from build123d import *

# Parameters (mm, degrees)
CROQUIS2_W              = 43
CROQUIS2_H              = 30
SALIENTE_EXTRUIR1_DEPTH = 30
CROQUIS3_W              = 42.529407755
CROQUIS3_H              = 25.558495791
CORTAR_EXTRUIR1_DEPTH   = 30
CORTAR_EXTRUIR2_START   = -7.5
CORTAR_EXTRUIR2_DEPTH   = 15
CORTAR_EXTRUIR4_DEPTH   = 4.5
CORTAR_EXTRUIR5_DEPTH   = 4.5
REDONDEO1_R             = 3
CROQUIS8_W              = 15
CROQUIS8_H              = 32.397186909
CORTAR_EXTRUIR6_DEPTH   = 4.5
CROQUIS9_W              = 120.283196461
CROQUIS9_H              = 78.810135234
CORTAR_EXTRUIR7_DEPTH   = 22.5


with BuildPart() as part:
    # Croquis2 → Saliente-Extruir1 (new body)
    with BuildSketch(Plane(origin=(0, 0, 0), x_dir=(0, 0, -1), z_dir=(1, 0, 0))):
        with Locations((-19.783269962, -13.522813688)):
            Rectangle(CROQUIS2_W, CROQUIS2_H)
    extrude(amount=SALIENTE_EXTRUIR1_DEPTH)

    # Croquis3 → Cortar-Extruir1 (cut)
    with BuildSketch(Plane(origin=(30, 0, 0), x_dir=(0, 0, -1), z_dir=(1, 0, 0))):
        with Locations((-17.018566085, -31.302061584)):
            Rectangle(CROQUIS3_W, CROQUIS3_H)
        Polygon((-31.675073764, 1.477186312), (-3.283269962, -16.522813688), (1.716730038, -16.522813688), (1.716730038, 1.477186312), align=None)
    extrude(amount=-CORTAR_EXTRUIR1_DEPTH, mode=Mode.SUBTRACT)

    # Croquis4 → Cortar-Extruir2 (cut)
    with BuildSketch(Plane(origin=(30, 0, 0), x_dir=(0, 0, -1), z_dir=(1, 0, 0)).offset(CORTAR_EXTRUIR2_START)):
        Polygon((-41.283269962, -1.522813688), (-32.545919554, -1.522813688), (-8.886083053, -16.522813688), (-41.283269962, -16.522813688), align=None)
    extrude(amount=-CORTAR_EXTRUIR2_DEPTH, mode=Mode.SUBTRACT)

    # Croquis5 → Cortar-Extruir4 (cut)
    with BuildSketch(Plane(origin=(30, 0, 0), x_dir=(0, 0, -1), z_dir=(1, 0, 0))):
        Polygon((-3.283269962, -16.522813688), (-41.283269962, -16.522813688), (-41.283269962, 1.477186312), (-31.675073764, 1.477186312), align=None)
    extrude(amount=-CORTAR_EXTRUIR4_DEPTH, mode=Mode.SUBTRACT)

    # Croquis6 → Cortar-Extruir5 (cut)
    with BuildSketch(Plane.ZY):
        Polygon((3.283269962, -16.522813688), (41.283269962, -16.522813688), (41.283269962, 1.477186312), (31.675073764, 1.477186312), align=None)
    extrude(amount=-CORTAR_EXTRUIR5_DEPTH, mode=Mode.SUBTRACT)

    # Redondeo1
    redondeo1_edges = [part.edges().sort_by_distance(p)[0] for p in [
        (0, -17.522813688, -1.716730038),
        (30, -17.522813688, -1.716730038),
    ]]
    fillet(redondeo1_edges, radius=REDONDEO1_R)

    # Croquis8 → Cortar-Extruir6 (cut)
    with BuildSketch(Plane(origin=(0, -16.522813688, 0), x_dir=(1, 0, 0), z_dir=(0, 1, 0))):
        with Locations((15, -25.084676508)):
            Rectangle(CROQUIS8_W, CROQUIS8_H)
    extrude(amount=-CORTAR_EXTRUIR6_DEPTH, mode=Mode.SUBTRACT)

    # Croquis9 → Cortar-Extruir7 (cut)
    with BuildSketch(Plane.XZ.offset(18.522813688)):
        with Locations((17.6156444, 62.089659259)):
            Rectangle(CROQUIS9_W, CROQUIS9_H)
    extrude(amount=CORTAR_EXTRUIR7_DEPTH, mode=Mode.SUBTRACT)


solid = part.part
Geometry: final body of the model. Coordinates: model frame, mm. A direction names the side the tool comes from. Give positions to 0.01 mm unless a question says otherwise; leave off trailing zeros. Write each loop counter-clockwise with the first axis right and the second up, starting at its lowest first coordinate (ties: lowest second). Pieces come first, ordered by that corner, then holes. Notation, with made-up numbers: M 39.25,15 L 86.25,15 A18 cw 86.25,42 Z; hole C 29,2.5 d4. An arc over 180 degrees is marked long. Answer in a Markdown table with one row per item. Add a question column.
(1) Section C-C on z = 39.5. Return loops of the section in (x, y).
(2) Ray query, line 1 (X direction, y = -6.75, z = 34.5); line 2 (Y direction, x = 2.25, z = 1); line 3 (X direction, y = -4.5, z = 24). Return the intervals inside material, ascending.
(3) Section D-D on x = 6.5. Return loops of the section in (y, z).
(4) Reachability of faces 5 (the flat face through (25.5, -9, 26)), 6 (the flat face through (7.5, -12, 29)), 7 (the flat face through (4, -16.523, 15)), 8 (the flat face through (4.5, -9, 26)) from +Z, -Z, +X, -X, +Y, -Y: full face, straight path, thin tool, end or side. Return the list, or none.
(5) Section B-B on y = -10.5. Return loops of the section in (x, z), and give its area (3 significant figures).
(6) Mould query, pull axis X, two halves, no side actions, for faces 1 (the flat face through (15, -1.523, 37)), 2 (the flat face through (16, -1, 41.283)), 3 (the flat face through (30, -18, 22)), 4 (the flat face through (0, -18, 22)). Classes: +X half, -X half, draft (parallel to the pull), parting line (faces both ways), or undercut.
(7) First-contact query: pin 1 (8.5 mm diameter, centred on y = -11.5, z = 27, fed in from -X); pin 2 (1.5 mm diameter, centred on x = 11, y = -16, fed in from -Z); pin 3 (1.5 mm diameter, centred on x = 9.5, y = -14.5, fed in from +Z); pin 4 (2.5 mm diameter, centred on x = 13, z = 38, fed in from -Y). Flat tips, straight axial feed; report the tip coordinate or a pass-through.
(8) Section A-A on x = 12. Return loops of the section in (y, z), and give its area (3 significant figures).
Result set:
| question | item | result |
|---|---|---|
| 1 | outline | M 0,-18.52 L 7.5,-18.52 L 7.5,-1.52 L 22.5,-1.52 L 22.5,-18.52 L 30,-18.52 L 30,-16.52 L 25.5,-16.52 L 25.5,1.48 L 4.5,1.48 L 4.5,-16.52 L 0,-16.52 Z |
| 2 | line 1 | x = 4.5 to 7.5, 22.5 to 25.5 |
| 2 | line 2 | y = -18.52 to -16.52 |
| 2 | line 3 | x = 4.5 to 25.5 |
| 3 | outline | M -18.52,-1.72 L -16.52,-1.72 L -16.52,3.28 L 1.48,31.68 L 1.48,41.28 L -18.52,41.28 Z |
| 4 | face 5 | +Z, -Z, +X, +Y |
| 4 | face 6 | +Z, -Y |
| 4 | face 7 | -Z, +Y |
| 4 | face 8 | +Z, -Z, -X, +Y |
| 5 | outline | M 4.5,12.78 L 25.5,12.78 L 25.5,41.28 L 22.5,41.28 L 22.5,18.39 L 7.5,18.39 L 7.5,41.28 L 4.5,41.28 Z |
| 5 | area | 255 mm^2 |
| 6 | face 1 | undercut |
| 6 | face 2 | draft |
| 6 | face 3 | +X half |
| 6 | face 4 | -X half |
| 7 | pin 1 | stops at x = 4.5 |
| 7 | pin 2 | stops at z = -1.72 |
| 7 | pin 3 | stops at z = 13.26 |
| 7 | pin 4 | stops at y = -1.52 |
| 8 | outline | M -18.52,-1.72 L -16.52,-1.72 L -16.52,3.28 L 1.48,31.68 L 1.48,41.28 L -1.52,41.28 L -1.52,32.55 L -16.52,8.89 L -18.52,8.89 Z |
| 8 | area | 141 mm^2 |
